```python
from build123d import *

# Parameters (mm, degrees)
SKETCH_1_R          = 3.5
EXTRUDE_1_DEPTH     = 3.1
EXTRUDE_2_DEPTH     = 1.2
SKETCH_3_R          = 1.5
CUT_EXTRUDE_1_DEPTH = 3
CUT_EXTRUDE_2_REACH = 18.974
SKETCH_4_R          = 0.5


with BuildPart() as part:
    # Sketch 1 → Extrude 1 (new body)
    with BuildSketch(Plane(origin=(0, 0, 0), x_dir=(1, 0, 0), z_dir=(0, 1, 0))):
        with Locations(Location((0, 0, 0), (0, 0, 90))):
            Circle(SKETCH_1_R)
    extrude(amount=EXTRUDE_1_DEPTH)

    # Sketch 2 → Extrude 2 (add)
    with BuildSketch(Plane(origin=(0, 0, 0), x_dir=(1, 0, 0), z_dir=(0, 1, 0))):
        with BuildLine():
            Line((-3, -1.802775638), (-2, -14.5))
            ThreePointArc((-2, -14.5), (0, -16.5), (2, -14.5))
            Line((2, -14.5), (3, -1.802775638))
            ThreePointArc((3, -1.802775638), (0, -3.5), (-3, -1.802775638))
        make_face()
    extrude(amount=EXTRUDE_2_DEPTH)

    # Sketch 3 → Cut-Extrude 1 (cut)
    with BuildSketch(Plane(origin=(0, 3.1, 0), x_dir=(1, 0, 0), z_dir=(0, 1, 0))):
        with Locations(Location((0, 0, 0), (0, 0, 270))):
            Circle(SKETCH_3_R)
    extrude(amount=-CUT_EXTRUDE_1_DEPTH, mode=Mode.SUBTRACT)

    # Sketch 4 → Cut-Extrude 2 (cut, up to next)
    with BuildSketch(Plane(origin=(0, 1.2, 0), x_dir=(1, 0, 0), z_dir=(0, 1, 0)), mode=Mode.PRIVATE) as cut_extrude_2_sk1:
        with Locations(Location((0, -14.5, 0), (0, 0, 270))):
            Circle(SKETCH_4_R)
    cut_extrude_2_tool1 = extrude(cut_extrude_2_sk1.sketch, amount=-CUT_EXTRUDE_2_REACH, mode=Mode.PRIVATE) & part.part
    # Sketch 4 → Cut-Extrude 2 (cut, up to next)
    with BuildSketch(Plane(origin=(0, 1.2, 0), x_dir=(1, 0, 0), z_dir=(0, 1, 0)), mode=Mode.PRIVATE) as cut_extrude_2_sk2:
        with Locations(Location((0, -12, 0), (0, 0, 270))):
            Circle(SKETCH_4_R)
    cut_extrude_2_tool2 = extrude(cut_extrude_2_sk2.sketch, amount=-CUT_EXTRUDE_2_REACH, mode=Mode.PRIVATE) & part.part
    # Sketch 4 → Cut-Extrude 2 (cut, up to next)
    with BuildSketch(Plane(origin=(0, 1.2, 0), x_dir=(1, 0, 0), z_dir=(0, 1, 0)), mode=Mode.PRIVATE) as cut_extrude_2_sk3:
        with Locations(Location((0, -9.5, 0), (0, 0, 270))):
            Circle(SKETCH_4_R)
    cut_extrude_2_tool3 = extrude(cut_extrude_2_sk3.sketch, amount=-CUT_EXTRUDE_2_REACH, mode=Mode.PRIVATE) & part.part
    # Sketch 4 → Cut-Extrude 2 (cut, up to next)
    with BuildSketch(Plane(origin=(0, 1.2, 0), x_dir=(1, 0, 0), z_dir=(0, 1, 0)), mode=Mode.PRIVATE) as cut_extrude_2_sk4:
        with Locations(Location((0, -7, 0), (0, 0, 270))):
            Circle(SKETCH_4_R)
    cut_extrude_2_tool4 = extrude(cut_extrude_2_sk4.sketch, amount=-CUT_EXTRUDE_2_REACH, mode=Mode.PRIVATE) & part.part
    # Sketch 4 → Cut-Extrude 2 (cut, up to next)
    with BuildSketch(Plane(origin=(0, 1.2, 0), x_dir=(1, 0, 0), z_dir=(0, 1, 0)), mode=Mode.PRIVATE) as cut_extrude_2_sk5:
        with Locations(Location((0, -4.5, 0), (0, 0, 270))):
            Circle(SKETCH_4_R)
    cut_extrude_2_tool5 = extrude(cut_extrude_2_sk5.sketch, amount=-CUT_EXTRUDE_2_REACH, mode=Mode.PRIVATE) & part.part
    add(cut_extrude_2_tool1.solids().sort_by_distance((0, 1.2, 14.5))[0], mode=Mode.SUBTRACT)
    add(cut_extrude_2_tool2.solids().sort_by_distance((0, 1.2, 12))[0], mode=Mode.SUBTRACT)
    add(cut_extrude_2_tool3.solids().sort_by_distance((0, 1.2, 9.5))[0], mode=Mode.SUBTRACT)
    add(cut_extrude_2_tool4.solids().sort_by_distance((0, 1.2, 7))[0], mode=Mode.SUBTRACT)
    add(cut_extrude_2_tool5.solids().sort_by_distance((0, 1.2, 4.5))[0], mode=Mode.SUBTRACT)


solid = part.part
```
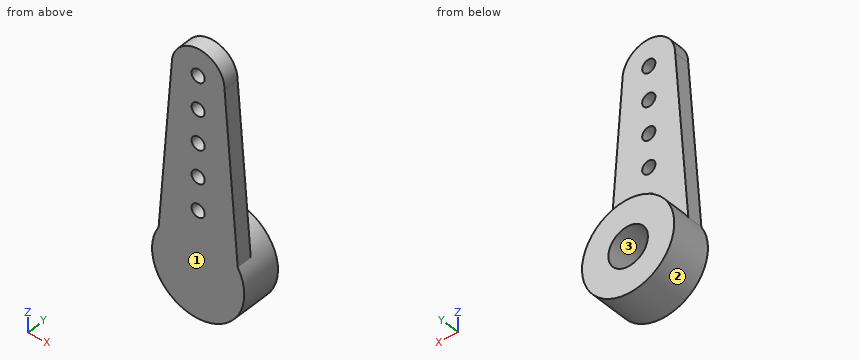
Geometry check sheet. Reference: the model listing, model coordinates, mm. Face numbers are marked on the shaded views. Coordinates: 2 decimals unless noted, no trailing zeros. Loops run counter-clockwise (first coordinate to the right, second up) from the corner with the lowest first, then second, coordinate; pieces in that order, holes last. Notation, with made-up numbers: (89.5, -22) - (125.5, -22) arc R17 ccw to (125.5, -15) - close; hole circle Ø2 at (-38.5, 81.25). An arc over 180 degrees is marked (long way). One line per item, written item: value. Start each with the question number.
(1) Cross-section at D-D on z = 4.5. Enter the section's corners in (x, y).
(2) Material ranges on line 1 (Y direction, x = -2.5, z = 5.75); line 2 (Z direction, x = 0.5, y = 1.85); line 3 (Z direction, x = -1, y = 1.3), recorded low to high. Write a range as [from, to].
(3) Cross-section at B-B on x = 0. Count the separate pieces of the cut face and the enclosed holes in it, plus the area to 3 significant figures.
(4) Mould release check, pull along X, two halves, no side actions. Record for the marked faces 1, 2 and 3: released by +X, released by -X, zero draft, split by the parting line, or undercut.
(5) Cross-section at A-A on y = 0.8. Enter the section's corners in (x, z).
(6) Cross-section at C-C on z = 0. Enter the section's corners in (x, y).
(7) Depth check by flat-ended pin: P1, Ø0.9, axis at x = -0.5, z = 0, coming from the +Y side; P2, Ø4, axis at x = 1.5, z = 6.5, coming from the +Y side; P3, Ø4, axis at x = 0, z = 0, coming from the +Y side. Enter the tip coordinate at first touch or a pass-through.
Results below:
1. outline: (-2.79, 0) - (-0.5, 0) - (-0.5, 1.2) - (-2.79, 1.2) - close; (0.5, 0) - (2.79, 0) - (2.79, 1.2) - (0.5, 1.2) - close
2. line 1: y = [0, 1.2]
2. line 2: z = [-3.46, -1.41], [1.41, 3.46]
2. line 3: z = [-3.35, -1.12], [1.12, 3.35]
3. separate pieces: 6
3. enclosed holes: 0
3. area: 22.3 mm2
4. face 1: zero draft
4. face 2: split by the parting line
4. face 3: undercut
5. outline: (-3, 1.8) arc R3.5 ccw (long way) to (3, 1.8) - (2, 14.5) arc R2 ccw to (-2, 14.5) - close; hole circle Ø3 at (0, 0); hole circle Ø1 at (0, 4.5); hole circle Ø1 at (0, 7); hole circle Ø1 at (0, 9.5); hole circle Ø1 at (0, 12); hole circle Ø1 at (0, 14.5)
6. outline: (-3.5, 0) - (3.5, 0) - (3.5, 3.1) - (1.5, 3.1) - (1.5, 0.1) - (-1.5, 0.1) - (-1.5, 3.1) - (-3.5, 3.1) - close
7. P1: stops at y = 0.1
7. P2: stops at y = 1.2
7. P3: stops at y = 3.1
